```python
from build123d import *

# Parameters (mm, degrees)
SKETCH1_R                = 40
SKETCH1_R_2              = 30
BOSS_EXTRUDE1_DEPTH      = 70
SKETCH2_R                = 30
BOSS_EXTRUDE2_DEPTH      = 119
BOSS_EXTRUDE2_DEPTH_BACK = 10
CUT_EXTRUDE1_DEPTH       = 20
SKETCH5_R                = 10
CUT_EXTRUDE2_DEPTH       = 55


with BuildPart() as part:
    # Sketch1 → Boss-Extrude1 (new body)
    with BuildSketch(Plane.XY):
        Circle(SKETCH1_R)
        Circle(SKETCH1_R_2, mode=Mode.SUBTRACT)
    extrude(amount=-BOSS_EXTRUDE1_DEPTH)

    # Sketch2 → Boss-Extrude2 (add, two sides)
    with BuildSketch(Plane(origin=(0, 0, -70), x_dir=(-1, 0, 0), z_dir=(0, 0, -1))) as boss_extrude2_sk:
        Circle(SKETCH2_R)
    extrude(amount=BOSS_EXTRUDE2_DEPTH)
    extrude(boss_extrude2_sk.sketch, amount=-BOSS_EXTRUDE2_DEPTH_BACK)

    # Sketch4 → Cut-Extrude1 (cut)
    with BuildSketch(Plane(origin=(0, 0, -189), x_dir=(-1, 0, 0), z_dir=(0, 0, -1))):
        Polygon((8.5, -14.722431864), (17, 0), (8.5, 14.722431864), (-8.5, 14.722431864), (-17, 0), (-8.5, -14.722431864), align=None)
    extrude(amount=-CUT_EXTRUDE1_DEPTH, mode=Mode.SUBTRACT)

    # Sketch5 → Cut-Extrude2 (cut, symmetric)
    with BuildSketch(Plane(origin=(0, 0, 0), x_dir=(0, 0, -1), z_dir=(1, 0, 0))):
        with Locations((35, 0)):
            Circle(SKETCH5_R)
    extrude(amount=CUT_EXTRUDE2_DEPTH, both=True, mode=Mode.SUBTRACT)


solid = part.part
```
Verification items for the finished model (mm, model axes). A direction names the side the tool comes from. Round coordinates to 2 decimals unless told otherwise and drop trailing zeros. Order: outer loops, then holes, each group sorted by start corner. A loop starts at its lowest first (then second) coordinate and runs counter-clockwise, first axis right, second up. Notation, with made-up numbers: (-19.5, 69.5) - (-1.5, 69.5) arc R30 cw to (-1.5, 100.5) - close; hole circle Ø4 at (75.25, 84). An arc over 180 degrees is marked (long way). Use CSV: the item, a comma, the result in double quotes. Start each with the question number.
1) Section check D-D, the plane x = 0. Record the cut outline in (y, z).
2) Go/stop test with flat-tipped pins: P1, Ø8, axis at x = -5.5, z = -38, coming from the -Y side; P2, Ø8.5, axis at x = -3.5, z = -179.5, coming from the +Y side; P3, Ø8.5, axis at x = -0.5, z = -177.5, coming from the -Y side. Record where each tip stops, or that it passes through.
3) Section check C-C, the plane z = -19.5. Record the cut outline in (x, y), plus the area to 3 significant figures.
4) Section check B-B, the plane x = 24. Record the cut outline in (y, z).
5) Section check A-A, the plane z = -40. Record the cut outline in (x, y), plus the area to 3 significant figures.
6) Mould release check, pull along Z, two halves, no side actions. Record for faces 1 (the flat face through (6, 30, 0)), 2 (the cylindrical face through (-34.06, 3, -44.54)), 3 (the flat face through (6, 30, -70)): +Z half, -Z half, draft (parallel to the pull), parting line (faces both ways), or undercut.
7) Access from +Z, -Z, +X, -X, +Y, -Y to the whole of each face (thin tool, end or side, straight path). Record for faces 4 (the cylindrical face through (27.712, -11.49, -29.58)), 5 (the flat face through (-12.81, 7.26, -179.14)), 6 (the cylindrical face through (34.224, -3.83, -44.237)).
8) Thickness scan on L1, parallel to Y at x = 0, z = -43; L2, parallel to Z at x = 31.5, y = 0; L3, parallel to X at y = -7, z = -42.5. Record the ranges inside material, lowest first.
Answers:
1,outline,"(-40, -70) - (-30, -70) - (-30, -189) - (-14.72, -189) - (-14.72, -169) - (14.72, -169) - (14.72, -189) - (30, -189) - (30, -70) - (40, -70) - (40, 0) - (30, 0) - (30, -60) - (-30, -60) - (-30, 0) - (-40, 0) - close"
2,P1,"stops at y = -39.97"
2,P2,"stops at y = 30"
2,P3,"stops at y = -30"
3,outline,"circle Ø80 at (0, 0); hole circle Ø60 at (0, 0)"
3,area,"2,200 mm²"
4,outline,"(-32, -70) - (-18, -70) - (-18, -189) - (18, -189) - (18, -70) - (32, -70) - (32, 0) - (18, 0) - (18, -60) - (-18, -60) - (-18, 0) - (-32, 0) - close"
5,outline,"(-39.05, -8.66) arc R40 ccw to (39.05, -8.66) - (28.72, -8.66) arc R30 cw to (-28.72, -8.66) - close; (-39.05, 8.66) - (-28.72, 8.66) arc R30 cw to (28.72, 8.66) - (39.05, 8.66) arc R40 ccw to start"
5,area,"1,850 mm²"
6,face 1,"+Z half"
6,face 2,"undercut"
6,face 3,"-Z half"
7,face 4,"+Z"
7,face 5,"-Z"
7,face 6,"+X, -X"
8,L1,"y = -40 to -30, 30 to 40"
8,L2,"z = -70 to -45, -25 to 0"
8,L3,"x = -39.38 to -29.17, 29.17 to 39.38"
